Geometry: final body of the model. Coordinates: model frame, mm. A direction names the side the tool comes from. Round coordinates to 2 decimals unless told otherwise and drop trailing zeros. Loops run counter-clockwise (first coordinate to the right, second up) from the corner with the lowest first, then second, coordinate; pieces in that order, holes last. Notation, with made-up numbers: (-20.75, -30) -> (-5.75, -30) arc R16 ccw to (-5.75, -13) -> close; hole circle Ø9 at (63, -16.75). An arc over 180 degrees is marked (long way). Answer in a Markdown table with one row per item.
```python
from build123d import *

# Parameters (mm, degrees)
BOSS_EXTRUDE1_DEPTH = 4
SKETCH2_R           = 1
CUT_EXTRUDE1_DEPTH  = 10.581883948
SKETCH3_R           = 1
CUT_EXTRUDE2_DEPTH  = 10.581883948
FILLET1_R           = 1


with BuildPart() as part:
    # Sketch1 → Boss-Extrude1 (new body)
    with BuildSketch(Plane(origin=(0, 0, 0), x_dir=(0, 0, -1), z_dir=(1, 0, 0))):
        Polygon((0, 0), (0, 6.75), (-2, 6.75), (-2, -2), (5.5, -2), (5.5, 0), align=None)
    extrude(amount=BOSS_EXTRUDE1_DEPTH)

    # Sketch2 → Cut-Extrude1 (cut, through all)
    with BuildSketch(Plane(origin=(0, 0, 0), x_dir=(-1, 0, 0), z_dir=(0, 0, -1))):
        with Locations(Location((-2, 4, 0), (0, 0, 90))):
            Circle(SKETCH2_R)
    extrude(amount=-CUT_EXTRUDE1_DEPTH, mode=Mode.SUBTRACT)

    # Sketch3 → Cut-Extrude2 (cut, through all)
    with BuildSketch(Plane(origin=(0, 0, 0), x_dir=(1, 0, 0), z_dir=(0, 1, 0))):
        with Locations(Location((2, 3, 0), (0, 0, 270))):
            Circle(SKETCH3_R)
    extrude(amount=-CUT_EXTRUDE2_DEPTH, mode=Mode.SUBTRACT)

    # Fillet1
    fillet1_edges = [part.edges().sort_by_distance(p)[0] for p in [
        (2, 0, 0),
    ]]
    fillet(fillet1_edges, radius=FILLET1_R)


solid = part.part
```
Item 1: Section query D-D, the plane z = 0.75. Output: boundary loops of the cut face in (x, y).
Ans:
| item | result |
|---|---|
| outline | (0, -2) -> (4, -2) -> (4, 6.75) -> (0, 6.75) -> close; hole circle Ø2 at (2, 4) |
Item 2: Ray query, L1, parallel to X at y = -1.2, z = -3; L2, parallel to Y at x = 3, z = -3.5; L3, parallel to Y at x = 2.3, z = 1.25. Return the intervals inside material, ascending.
Ans:
| item | result |
|---|---|
| L1 | 0 to 1, 3 to 4 |
| L2 | -2 to 0 |
| L3 | -2 to 3.05, 4.95 to 6.75 |
Item 3: Mould query, pull axis X, two halves, no side actions, for faces 1 (the cylindrical face through (1.4, -1, -3.8)), 2 (the flat face through (0, 0, 0)), 3 (the flat face through (2, 6.75, 1)), 4 (the cylindrical face through (1.4, 3.2, 1)). Classes: released by +X, released by -X, zero draft, split by the parting line, or undercut.
Ans:
| item | result |
|---|---|
| face 1 | undercut |
| face 2 | released by -X |
| face 3 | zero draft |
| face 4 | undercut |
Item 4: Set-up query: faces 5 (the flat face through (2, 0, -4.3)), 6 (the flat face through (2, -2, -1.7)). Return all of +Z, -Z, +X, -X, +Y, -Y with unobstructed straight access to the full face (end or side cutting, diameter ignored); none if empty.
Ans:
| item | result |
|---|---|
| face 5 | -Z, +X, -X, +Y |
| face 6 | +Z, -Z, +X, -X, -Y |
Item 5: First-contact query: P1, Ø2, axis at x = 3, z = -4, coming from the +Y side. Flat tip, straight axial feed; report the tip coordinate or a pass-through.
Ans:
| item | result |
|---|---|
| P1 | y = 0 |
Item 6: Section query C-C, the plane x = 2. Output: boundary loops of the cut face in (y, z).
Ans:
| item | result |
|---|---|
| outline | (-2, -5.5) -> (0, -5.5) -> (0, -4) -> (-2, -4) -> close; (-2, -2) -> (0, -2) -> (0, -1) arc R1 cw to (1, 0) -> (3, 0) -> (3, 2) -> (-2, 2) -> close; (5, 0) -> (6.75, 0) -> (6.75, 2) -> (5, 2) -> close |
Item 7: Section query B-B, the plane z = -3. Output: boundary loops of the cut face in (x, y).
Ans:
| item | result |
|---|---|
| outline | (0, -2) -> (1, -2) -> (1, 0) -> (0, 0) -> close; (3, -2) -> (4, -2) -> (4, 0) -> (3, 0) -> close |
Item 8: Section query A-A, the plane y = 4. Output: boundary loops of the cut face in (x, z), and give its area (3 significant figures).
Ans:
| item | result |
|---|---|
| outline | (0, 0) -> (1, 0) -> (1, 2) -> (0, 2) -> close; (3, 0) -> (4, 0) -> (4, 2) -> (3, 2) -> close |
| area | 4.00 mm2 |
